CAD build for the part. Positions are in the model's coordinates, mm. A direction names the side the tool comes from. Coordinates: 2 decimals unless noted, no trailing zeros. Order: outer loops, then holes, each group sorted by start corner. A loop starts at its lowest first (then second) coordinate and runs counter-clockwise, first axis right, second up. Notation, with made-up numbers: M 26,55 L 42,55 A22 ccw 42,68 Z; hole C -29.5,40.5 d8. An arc over 180 degrees is marked long. One line per item, written item: value.
from build123d import *

# Parameters (mm, degrees)
F0_R     = 25.4
F1_DEPTH = 25.4
F2_R     = 25.39999
F3_R     = 12.7
F4_DEPTH = 12.7
F5_R     = 12.7
F6_DEPTH = 12.7


# Not quite as in the source:
# - a fillet or chamfer is up to 0.001 mm smaller than in the source, because OpenCascade refuses the exact size


with BuildPart() as f1:
    # F0 (on Front) → F1 (new body, symmetric)
    with BuildSketch(Plane.XZ):
        with BuildLine():
            ThreePointArc((12.7, -35.9210244843), (31.1085197333, -21.9970452561), (38.1, 0))
            ThreePointArc((38.1, 0), (-21.9970452561, 31.1085197333), (-12.7, -35.9210244843))
            ThreePointArc((-12.7, -35.9210244843), (0, -38.1), (12.7, -35.9210244843))
        make_face()
        Circle(F0_R, mode=Mode.SUBTRACT)
        with BuildLine():
            ThreePointArc((12.7, -35.9210244843), (0, -38.1), (-12.7, -35.9210244843))
            Line((-12.7, -35.9210244843), (-12.7, -203.2))
            Line((-12.7, -203.2), (-38.1, -203.2))
            Line((-38.1, -203.2), (-38.1, -292.1))
            Line((-38.1, -292.1), (-25.4, -292.1))
            Line((-25.4, -292.1), (-25.4, -215.9))
            Line((-25.4, -215.9), (25.4, -215.9))
            Line((25.4, -215.9), (25.4, -292.1))
            Line((25.4, -292.1), (38.1, -292.1))
            Line((38.1, -292.1), (38.1, -203.2))
            Line((38.1, -203.2), (12.7, -203.2))
            Line((12.7, -203.2), (12.7, -35.9210244843))
        make_face()
    extrude(amount=F1_DEPTH, both=True)

    # F2 (radius 25.4 in the source; OpenCascade refuses exactly that, so slightly less here)
    f2_edges = [f1.edges().sort_by_distance(p)[0] for p in [
        (12.7, 0, -35.921024),
        (-12.7, 0, -35.921024),
        (-31.75, -25.4, -292.1),
        (-31.75, 25.4, -292.1),
        (31.75, -25.4, -292.1),
        (31.75, 25.4, -292.1),
    ]]
    fillet(f2_edges, radius=F2_R)

    # F3 (on face) → F4 (cut, through all)
    with BuildSketch(Plane(origin=(-38.1, 0, 0), x_dir=(0, -1, 0), z_dir=(-1, 0, 0))):
        with Locations((0, -266.7)):
            Circle(F3_R)
    extrude(amount=-F4_DEPTH, mode=Mode.SUBTRACT)

    # F5 (on face) → F6 (cut, through all)
    with BuildSketch(Plane.YZ.offset(38.1)):
        with Locations((0, -266.7)):
            Circle(F5_R)
    extrude(amount=-F6_DEPTH, mode=Mode.SUBTRACT)


solid = f1.part
Q1. Drill centre lines: line 1 along X through (y, z) = (18, -242.5); line 2 along X through (y, z) = (-12.5, -130.5); line 3 along X through (y, z) = (-7.5, -30.5). Where is each one in solid material? Low to high.
Recorded:
line 1: x = -38.1 to -25.4, 25.4 to 38.1
line 2: x = -12.7 to 12.7
line 3: x = -22.83 to 22.83
Q2. Slice it at C-C (y = 8). List the corners of the cut face in (x, z).
Recorded:
outline: M -38.1,-290.81 L -25.4,-290.81 L -25.4,-276.56 L -38.1,-276.56 Z; M -38.1,-256.84 L -25.4,-256.84 L -25.4,-215.9 L 25.4,-215.9 L 25.4,-256.84 L 38.1,-256.84 L 38.1,-203.2 L 12.7,-203.2 L 12.7,-50.8 A25.4 cw 22.86,-30.48 A38.1 ccw long -22.86,-30.48 A25.4 cw -12.7,-50.8 L -12.7,-203.2 L -38.1,-203.2 Z; M 25.4,-290.81 L 38.1,-290.81 L 38.1,-276.56 L 25.4,-276.56 Z; hole C 0,0 d50.8
Q3. Pin check, flat tips, straight feed: pin 1 Ø1.5 at (y, z) = (-1, -82) entering from -X; pin 2 Ø2 at (x, y) = (-0.5, 11.5) entering from +Z; pin 3 Ø5 at (x, y) = (21, 9) entering from +Z; pin 4 Ø15 at (y, z) = (-0.5, -270.5) entering from -X. Stop position of each tip, or through.
Recorded:
pin 1: stops at x = -12.7
pin 2: stops at z = 38.1
pin 3: stops at z = 33.31
pin 4: passes through
Q4. Which spindle directions (+Z, -Z, +X, -X, +Y, -Y) get a long thin tool onto all of the face, cutting with end or side? Do faces 4 (the face through (-25.4, 0, -246)), 5 (the face through (-15.456, -0.356, -39.294)), 6 (the face through (12.7, 0, -128)), 7 (the face through (31.84, -17.76, -284.86)), 8 (the face through (1.332, -0.356, 38.077)). Say none if no direction does.
Recorded:
face 4: -Z, +Y, -Y
face 5: -X, +Y, -Y
face 6: +X, +Y, -Y
face 7: -Z, +X, -X, -Y
face 8: +Y, -Y
Q5. Slice it at B-B (z = -239). List the corners of the cut face in (x, y).
Recorded:
outline: M -38.1,-25.4 L -25.4,-25.4 L -25.4,25.4 L -38.1,25.4 Z; M 25.4,-25.4 L 38.1,-25.4 L 38.1,25.4 L 25.4,25.4 Z
Q6. Mould opens along X. For faces 1 (the face through (-5.506, 0.356, -24.796)), 2 (the face through (31.839, 6.827, -255.991)), 3 (the face through (-38.1, 0, -237)) say: released by +X, released by -X, zero draft, split by the parting line, or undercut.
Recorded:
face 1: undercut
face 2: zero draft
face 3: released by -X
Q7. Slice it at A-A (x = 0). List the corners of the cut face in (y, z), plus the area to 3 significant figures.
Recorded:
outline: M -25.4,-215.9 L 25.4,-215.9 L 25.4,-25.4 L -25.4,-25.4 Z; M -25.4,25.4 L 25.4,25.4 L 25.4,38.1 L -25.4,38.1 Z
area: 10,300 mm^2
Q8. Slice it at D-D (z = -92). List the corners of the cut face in (x, y).
Recorded:
outline: M -12.7,-25.4 L 12.7,-25.4 L 12.7,25.4 L -12.7,25.4 Z
